Geometry check sheet. Reference: drawing and pictorial views, mm from the part's lowest x, y, z. A direction names the side the tool comes from. Coordinates: 2 decimals unless noted, no trailing zeros. Write each loop counter-clockwise with the first axis right and the second up, starting at its lowest first coordinate (ties: lowest second). Pieces come first, ordered by that corner, then holes. Notation, with made-up numbers: (-28, 60) - (-3, 60) arc R24 ccw to (-3, 97) - close; hole circle Ø1 at (81, 58). An arc over 180 degrees is marked (long way). Answer as a JSON object with one key per item and string values. Group by question number.
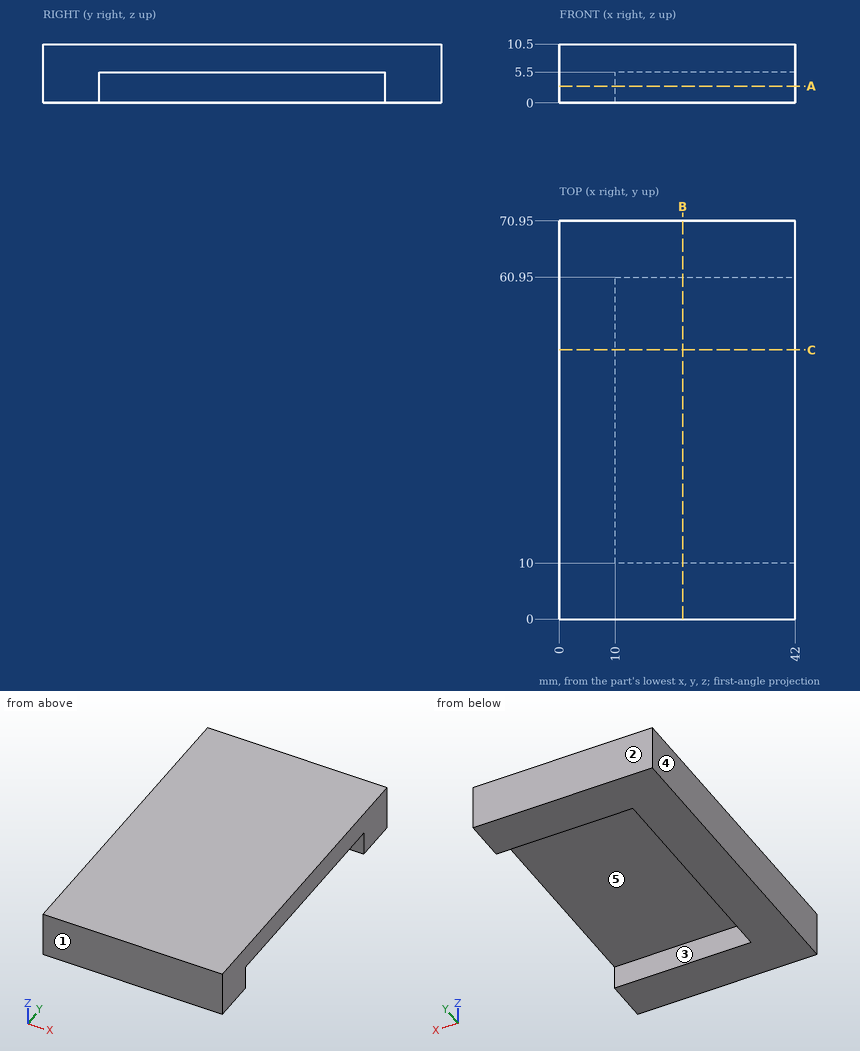
(1) Material ranges on L1, parallel to Y at x = 22.5, z = 4; L2, parallel to Z at x = 13, y = 57; L3, parallel to X at y = 54, z = 4.25, recorded low to high. Write a range as [from, to].
(2) Section check A-A (z = 3). Record the cut outline in (x, y).
(3) Draft check along Y on the marked faces 1, 2 and 3. Enter one of: +Y half, -Y half, draft (parallel to the pull), parting line (faces both ways), or undercut.
(4) Gauge pin test, flat ends, axial feed: pin 1 (2 mm diameter, centred on y = 41.5, z = 9, fed in from -X); pin 2 (4.5 mm diameter, centred on y = 47, z = 2.5, fed in from +X); pin 3 (3 mm diameter, centred on x = 25, y = 47.5, fed in from -Z). Record the tip position at first contact, or that the pin passes through.
(5) Section check C-C (y = 48). Record the cut outline in (x, z), and give its area (3 significant figures).
(6) Set-up check for the marked faces 4 and 5: record each of +Z, -Z, +X, -X, +Y, -Y from which the full face is reachable in a straight line by a thin tool's end or side.
(7) Section check B-B (x = 22). Record the cut outline in (y, z), and give its area (3 significant figures).
Conclusion:
{
 "1": {"L1": "y = [0, 10], [60.95, 70.95]", "L2": "z = [5.5, 10.5]", "L3": "x = [0, 10]"},
 "2": {"outline": "(0, 0) - (42, 0) - (42, 10) - (10, 10) - (10, 60.95) - (42, 60.95) - (42, 70.95) - (0, 70.95) - close"},
 "3": {"face 1": "-Y half", "face 2": "+Y half", "face 3": "undercut"},
 "4": {"pin 1": "stops at x = 0", "pin 2": "stops at x = 10", "pin 3": "stops at z = 5.5"},
 "5": {"outline": "(0, 0) - (10, 0) - (10, 5.5) - (42, 5.5) - (42, 10.5) - (0, 10.5) - close", "area": "265 mm^2"},
 "6": {"face 4": "+Z, -Z, -X, +Y, -Y", "face 5": "-Z, +X"},
 "7": {"outline": "(0, 0) - (10, 0) - (10, 5.5) - (60.95, 5.5) - (60.95, 0) - (70.95, 0) - (70.95, 10.5) - (0, 10.5) - close", "area": "465 mm^2"}
}
